Model file for the job. Use its own axes, mm. A direction names the side the tool comes from. Round coordinates to 2 decimals unless told otherwise and drop trailing zeros. Order: outer loops, then holes, each group sorted by start corner. A loop starts at its lowest first (then second) coordinate and runs counter-clockwise, first axis right, second up. Notation, with made-up numbers: (34.5, 55) -> (60.5, 55) arc R28 cw to (60.5, 75) -> close; hole circle Ø9 at (5, -19.75). An arc over 180 degrees is marked (long way). Put each result on its own line as item: value. Start each with the question number.
Q1. Flat gauge pins, fed straight in: P1, Ø2, axis at x = 4, z = -3, coming from the -Y side; P2, Ø3.5, axis at x = 1, z = 0, coming from the +Y side; P3, Ø1.2, axis at y = 7, z = -4.75, coming from the -X side. Where does each tip first touch, or does it go through?
Q2. Probe L1, parallel to Z at x = -11.95, y = 7; L2, parallel to X at y = 11.5, z = -0.25; L3, parallel to Z at x = 7, y = 2.75. List the from-to ranges inside material, lowest first.
Q3. Cut at B-B, the plane z = 4.75. List the corners of the cut face in (x, y).
Q4. 3-axis set-ups, long thin cutter, end or side, ignore diameter. For faces 4 (the face through (0, 3, -10.1)), 5 (the face through (-1.081, 12.972, 3.434)), 6 (the face through (-12.52, 6.01, -4.88)): which of +Z, -Z, +X, -X, +Y, -Y reach the whole face in a straight line?
Q5. Cut at C-C, the plane y = 11.5. List the corners of the cut face in (x, z), and give its area (3 significant figures).
Q6. Cut at D-D, the plane x = 5.25. List the corners of the cut face in (y, z).
Q7. Cut at A-A, the plane x = 0. List the corners of the cut face in (y, z), and give its area (3 significant figures).
Q8. Pull direction X, two halves, no side cores. Call faces 1 (the face through (-10.1, 7.4, -4.8)), 2 (the face through (10.1, 3, 0)), 3 (the face through (14.43, 7.6, -14.4)): released by +X, released by -X, zero draft, split by the parting line, or undercut.
Autodesk Inventor part; units mm, degrees
ref_plane "YZ Plane" through (0, 0, 0) normal (1, 0, 0) x (0, 1, 0)
ref_plane "XZ Plane" through (0, 0, 0) normal (0, 1, 0) x (-1, 0, 0)
ref_plane "XY Plane" through (0, 0, 0) normal (0, 0, 1) x (1, 0, 0)
sketch "草圖2" plane through (0, 0, 0) normal (0, 1, 0) x (-1, 0, 0)
  line L0 (-15, 15) -> (15, 15)
  line L1 (15, 15) -> (15, -15)
  line L2 (15, -15) -> (-15, -15)
  line L3 (-15, -15) -> (-15, 15)
  line L4 (-15, 15) -> (15, -15) construction
  line L5 (15, 15) -> (-15, -15) construction
  line L6 (-10.1, 10.1) -> (10.1, 10.1)
  line L7 (10.1, 10.1) -> (10.1, -10.1)
  line L8 (10.1, -10.1) -> (-10.1, -10.1)
  line L9 (-10.1, -10.1) -> (-10.1, 10.1)
  line L10 (-10.1, 10.1) -> (10.1, -10.1) construction
  line L11 (10.1, 10.1) -> (-10.1, -10.1) construction
  point P0 (0, 0)
  dimension "d4" = 30
  dimension "d5" = 30
  dimension "d6" = 20.2
  dimension "d7" = 20.2
extrude "擠出2" add sketch "草圖2" along normal blind 15
sketch "草圖3" plane through (0, 15, 0) normal (0, 1, 0) x (1, 0, 0)
  line L0 (15, 15) -> (-15, 15)
  line L1 (-15, 15) -> (-15, -15)
  line L2 (-15, -15) -> (15, -15)
  line L3 (15, -15) -> (15, 15)
  line L4 (10.1, -10.1) -> (-10.1, -10.1)
  line L5 (-10.1, -10.1) -> (-10.1, 10.1)
  line L6 (-10.1, 10.1) -> (10.1, 10.1)
  line L7 (10.1, 10.1) -> (10.1, -10.1)
  point P0 (0, 0)
extrude "擠出3" add sketch "草圖3" against normal blind 8 contours L4 L5 L6 L7
sketch "草圖4" plane through (0, 15, 0) normal (0, 1, 0) x (1, 0, 0)
  circle A0 centre (0, 0) radius 2.1
  dimension "d12" = 4.2
hole "孔1" at (0, 15, 0) direction (0, -1, 0) diameter 4.2 end through all counterbore diameter 7.2 counterbore depth 4
sketch "草圖5" plane through (-15, 0, -15) normal (-1, 0, 0) x (0, 0, 1)
  line L0 (10.25, 7) -> (19.75, 7) construction
  line L1 (0, 0) -> (30, 0) construction
  line L2 (0, 15) -> (30, 15) construction
  point P0 (15, 0)
  point P1 (15, 7)
  point P2 (15, 0)
  dimension "d20" = 9.5
  dimension "d21" = 8
hole "孔2" at (-15, 7, -4.75) at (-15, 7, 4.75) direction (1, 0, 0) diameter 2 depth 4.9
fillet "圓角1" radius 2 4 edges at (-15, 7.5, -15) (-15, 7.5, 15) (15, 7.5, -15) (15, 7.5, 15)
sketch "草圖1" plane through (0, 0, 0) normal (0, 1, 0) x (-1, 0, 0)
  line L0 (-10, 10) -> (10, 10)
  line L1 (10, 10) -> (10, -10)
  line L2 (10, -10) -> (-10, -10)
  line L3 (-10, -10) -> (-10, 10)
  line L4 (-10, 10) -> (10, -10) construction
  line L5 (10, 10) -> (-10, -10) construction
  point P0 (0, 0)
  dimension "d2" = 20
  dimension "d3" = 20
equation "\"d6\" = d7"
properties part number "限位開關"
Ans:
1. P1: stops at y = 7
1. P2: stops at y = 11
1. P3: stops at x = -10.1
2. L1: z = -15 to -5.75, -3.75 to 3.75, 5.75 to 15
2. L2: x = -15 to -3.59, 3.59 to 15
2. L3: z = -15 to -10.1, 10.1 to 15
3. outline: (-15, 0) -> (-10.1, 0) -> (-10.1, 6) -> (-15, 6) -> close; (-15, 8) -> (-10.1, 8) -> (-10.1, 7) -> (10.1, 7) -> (10.1, 0) -> (15, 0) -> (15, 15) -> (-15, 15) -> close
4. face 4: -Y
4. face 5: +Y
4. face 6: -X
5. outline: (-15, -13) arc R2 ccw to (-13, -15) -> (13, -15) arc R2 ccw to (15, -13) -> (15, 13) arc R2 ccw to (13, 15) -> (-13, 15) arc R2 ccw to (-15, 13) -> close; hole circle Ø7.2 at (0, 0)
5. area: 856 mm^2
6. outline: (0, -15) -> (15, -15) -> (15, 15) -> (0, 15) -> (0, 10.1) -> (7, 10.1) -> (7, -10.1) -> (0, -10.1) -> close
7. outline: (0, -15) -> (15, -15) -> (15, -3.6) -> (11, -3.6) -> (11, -2.1) -> (7, -2.1) -> (7, -10.1) -> (0, -10.1) -> close; (0, 10.1) -> (7, 10.1) -> (7, 2.1) -> (11, 2.1) -> (11, 3.6) -> (15, 3.6) -> (15, 15) -> (0, 15) -> close
7. area: 263 mm^2
8. face 1: released by -X
8. face 2: undercut
8. face 3: released by +X
